CAD build for the part. Positions are in the model's coordinates, mm. Face numbers are marked on the shaded views. A direction names the side the tool comes from. Round coordinates to 2 decimals unless told otherwise and drop trailing zeros. Write each loop counter-clockwise with the first axis right and the second up, starting at its lowest first coordinate (ties: lowest second). Pieces come first, ordered by that corner, then holes. Notation, with made-up numbers: M -21,28 L -4,28 A11 ccw -4,32 Z; hole C 53,19 d3. An arc over 180 degrees is marked long. Write each question's results on one line, items separated by ' | '. Start each with the question number.
```python
from build123d import *

# Parameters (mm, degrees)
F2_R = 5
F3_R = 10
F4_R = 5


with BuildPart() as f1:
    # F0 (on Front) → F1 (revolve)
    with BuildSketch(Plane.XZ):
        Polygon((55, 8), (93, 8), (93, 24.90327), (20, 44), (20, 55), (15, 60), (0, 60), (0, 28), (7, 28), (15, 14), (55, 14), align=None)
    revolve(axis=Axis((54.39201, 0, 0), (1, 0, 0)))

    # F2
    f2_edges = [f1.edges().sort_by_distance(p)[0] for p in [
        (93, 0, -24.90327),
    ]]
    fillet(f2_edges, radius=F2_R)

    # F3
    f3_edges = [f1.edges().sort_by_distance(p)[0] for p in [
        (20, 0, -44),
    ]]
    fillet(f3_edges, radius=F3_R)

    # F4
    f4_edges = [f1.edges().sort_by_distance(p)[0] for p in [
        (55, 0, -14),
    ]]
    fillet(f4_edges, radius=F4_R)


solid = f1.part
```
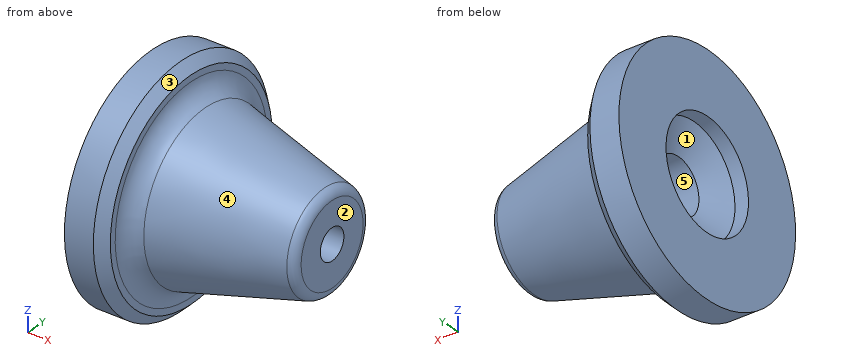
1) Drop flat-ended pins along their axis: pin 1 Ø1.5 at (y, z) = (37, -8) entering from -X; pin 2 Ø5 at (x, y) = (49, 3) entering from -Z; pin 3 Ø8 at (x, z) = (45, 12) entering from +Y; pin 4 Ø1.5 at (x, y) = (10, 40) entering from -Z. Give the stop position or say it passes through.
2) Saw through at A-A, the plane y = 0. Write the cut outline in (x, z), plus the area to 3 significant figures.
3) 3-axis set-ups, long thin cutter, end or side, ignore diameter. For the marked faces 4 and 5: which of +Z, -Z, +X, -X, +Y, -Y reach the whole face in a straight line?
4) Saw through at C-C, the plane x = 17. Write the cut outline in (y, z).
5) Saw through at D-D, the plane x = 34. Write the cut outline in (y, z).
6) Wall check: line 1 along X through (y, z) = (45, -25.5); line 2 along Y through (x, z) = (3.75, 0); line 3 along Z through (x, y) = (75, 0). Give the ranges that are in metal, low to high. Write a range as from..to.
7) Pull direction Z, two halves, no side cores. Call the marked faces 1, 2 and 3: pulls with the +Z half, pulls with the -Z half, needs draft (parallel to the pull), parting line crosses it, or undercut.
Filled sheet:
1) pin 1: stops at x = 0 | pin 2: stops at z = -36.97 | pin 3: stops at y = 37.08 | pin 4: stops at z = -45.38
2) outline: M 0,-60 L 15,-60 L 20,-55 L 20,-51.72 A10 cw 27.47,-42.05 L 89.27,-25.88 A5 ccw 93,-21.04 L 93,-8 L 55,-8 L 55,-9 A5 cw 50,-14 L 15,-14 L 7,-28 L 0,-28 Z; M 0,28 L 7,28 L 15,14 L 50,14 A5 cw 55,9 L 55,8 L 93,8 L 93,21.04 A5 ccw 89.27,25.88 L 27.47,42.05 A10 cw 20,51.72 L 20,55 L 15,60 L 0,60 Z | area: 4,980 mm^2
3) face 4: +X | face 5: -X
4) outline: C 0,0 d116; hole C 0,0 d28
5) outline: C 0,0 d80.68; hole C 0,0 d28
6) line 1: x = 0..20 | line 2: y = -60..-28, 28..60 | line 3: z = -29.61..-8, 8..29.61
7) face 1: undercut | face 2: needs draft | face 3: parting line crosses it
